```python
from build123d import *

# Parameters (mm, degrees)
F1_DEPTH = 8
F3_DEPTH = 10
F5_DEPTH = 9.9
F6_W     = 30.56961
F6_H     = 8
F7_DEPTH = 2
F6_R     = 1.3
F8_DEPTH = 6


with BuildPart() as f1:
    # F0 (on Top) → F1 (new body)
    with BuildSketch(Plane.XY):
        Polygon((28.5, -30), (-28.5, -30), (-36.985281, -21.514719), (-38.045942, -22.575379), (-30.62132, -30), (-33.166905, -32.545584), (-40.591526, -25.120963), (-41.652186, -26.181623), (-29.795584, -38.038225), (-28.312251, -32.5), (28.912205, -32.5), (29.795584, -38.038225), (41.652186, -26.181623), (40.591526, -25.120963), (33.166905, -32.545584), (30.62132, -30), (38.045942, -22.575379), (36.985281, -21.514719), align=None)
    extrude(amount=F1_DEPTH)

    # F2 (on face) → F3 (cut)
    with BuildSketch(Plane(origin=(33.916905, -33.916905, 0), x_dir=(0.707107, 0.707107, 0), z_dir=(0.707107, -0.707107, 0))):
        with BuildLine():
            ThreePointArc((7.671573, 4), (7.085786, 5.414214), (5.671573, 6))
            ThreePointArc((5.671573, 6), (3.671573, 4), (5.671573, 2))
            ThreePointArc((5.671573, 2), (7.085786, 2.585786), (7.671573, 4))
        make_face()
    extrude(amount=-F3_DEPTH, mode=Mode.SUBTRACT)

    # F4 (on face) → F5 (cut)
    with BuildSketch(Plane(origin=(-33.916905, -33.916905, 0), x_dir=(0.707107, -0.707107, 0), z_dir=(-0.707107, -0.707107, 0))):
        with BuildLine():
            ThreePointArc((-3.671573, 4), (-4.257359, 5.414214), (-5.671573, 6))
            ThreePointArc((-5.671573, 6), (-7.671573, 4), (-5.671573, 2))
            ThreePointArc((-5.671573, 2), (-4.257359, 2.585786), (-3.671573, 4))
        make_face()
    extrude(amount=-F5_DEPTH, mode=Mode.SUBTRACT)

    # F6 (on face) → F7 (join)
    with BuildSketch(Plane.XZ.offset(32.5)):
        with Locations((-2.027446, 4)):
            Rectangle(F6_W, F6_H)
    extrude(amount=F7_DEPTH)

    # F6 (on face) → F8 (join)
    with BuildSketch(Plane.XZ.offset(32.5)):
        with Locations((-25.312251, 2.5)):
            Circle(F6_R)
        with Locations((25.257359, 2.5)):
            Circle(F6_R)
    extrude(amount=F8_DEPTH)


solid = f1.part
```
Input: part model. Units: mm. Frame: model coordinates. A direction names the side the tool comes from. Coordinates: 2 decimals unless noted, no trailing zeros. Write each question's results on one line, items separated by ' | '.
Item 1: Set-up query: faces 4 (the flat face through (13.257, -33, 4)), 5 (the flat face through (-36, -29.71, 2.17)), 6 (the cylindrical face through (23.96, -35.46, 2.56)). Return all of +Z, -Z, +X, -X, +Y, -Y with unobstructed straight access to the full face (end or side cutting, diameter ignored); none if empty.
Conclusion:
face 4: +Z, -Z, -Y | face 5: +Z, -Z | face 6: -Y
Item 2: Mould query, pull axis Y, two halves, no side actions, for faces 1 (the flat face through (-17.312, -33, 4)), 2 (the flat face through (37.756, -27.956, 2.166)), 3 (the flat face through (-25, -38.5, 3)). Classes: +Y half, -Y half, draft (parallel to the pull), parting line (faces both ways), or undercut.
Conclusion:
face 1: draft | face 2: undercut | face 3: -Y half
Item 3: Material intervals for probe 1 along X at (y, z) = (-33.25, 4.25); probe 2 along X at (y, z) = (-25.25, 2.5); probe 3 along X at (y, z) = (-26, 7.75), sorted ascending.
Conclusion:
probe 1: x = -34.58 to -28.51, -17.31 to 13.26, 29.03 to 34.58 | probe 2: x = -40.72 to -40.46, -35.37 to -35.14, 35.14 to 35.37, 40.46 to 40.72 | probe 3: x = -41.47 to -39.71, -34.62 to -32.5, 32.5 to 34.62, 39.71 to 41.47
Item 4: Pin query (flat end, axial travel): pin 1 Ø4 at (x, z) = (5, 3.5) entering from -Y; pin 2 Ø2 at (y, z) = (-25, 1.5) entering from +X; pin 3 Ø1.6 at (y, z) = (-34, 3.5) entering from +X. Return the tip coordinate at first contact, or that it passes through.
Conclusion:
pin 1: stops at y = -34.5 | pin 2: stops at x = 41.47 | pin 3: stops at x = 34.63
